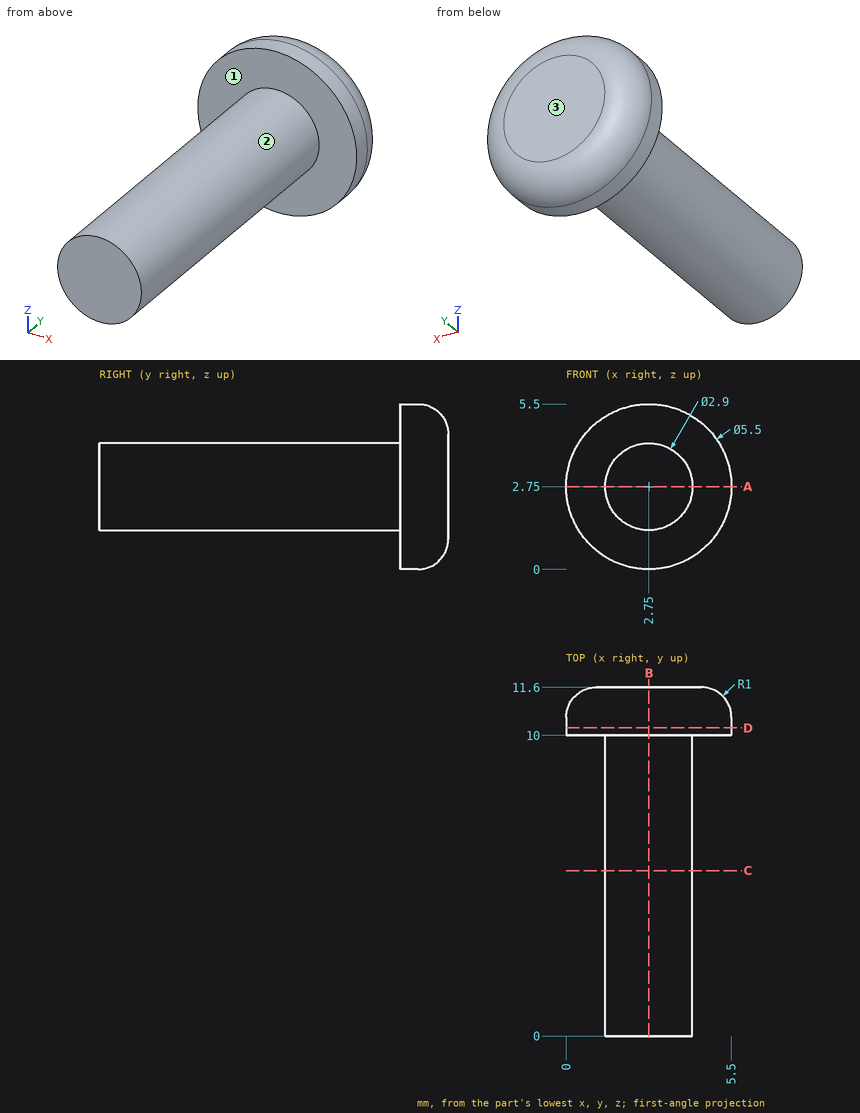
The figure shows three views and two pictorial views of one solid part (mm, origin at its lowest corner). Answer the questions. Give positions to 0.01 mm unless a question says otherwise; leave off trailing zeros. Loops run counter-clockwise (first coordinate to the right, second up) from the corner with the lowest first, then second, coordinate; pieces in that order, holes last. Notation, with made-up numbers: (76, 15.25) - (109, 15.25) arc R26 cw to (109, 52.25) - close; hole circle Ø6 at (35.25, 23.25). An arc over 180 degrees is marked (long way). Use one line per item in the form item = value.
1. Section D-D on y = 10.25 is taken. Give the vertices of the cut face in (x, z).
Calculated:
outline = circle Ø5.5 at (2.75, 2.75)
2. Section A-A on z = 2.75 is taken. Give the vertices of the cut face in (x, y).
Calculated:
outline = (0, 10) - (1.3, 10) - (1.3, 0) - (4.2, 0) - (4.2, 10) - (5.5, 10) - (5.5, 10.6) arc R1 ccw to (4.5, 11.6) - (1, 11.6) arc R1 ccw to (0, 10.6) - close
3. The mould has two halves that part along Y. Classify the marked faces 1, 2 and 3: pulls with the +Y half, pulls with the -Y half, needs draft (parallel to the pull), parting line crosses it, or undercut.
Calculated:
face_1 = pulls with the -Y half
face_2 = needs draft
face_3 = pulls with the +Y half
4. Find the intervals of material crossed by line 1 along X through (y, z) = (0.5, 3.45); line 2 along X through (y, z) = (10.5, 3.8); line 3 along Z through (x, y) = (1.85, 10.25), in increasing order. Write a range as [from, to].
Calculated:
line_1 = [1.48, 4.02]
line_2 = [0.21, 5.29]
line_3 = [0.15, 5.35]
5. Section B-B on x = 2.75 is taken. Give the vertices of the cut face in (y, z), then the cut area to 3 significant figures.
Calculated:
outline = (0, 1.3) - (10, 1.3) - (10, 0) - (10.6, 0) arc R1 ccw to (11.6, 1) - (11.6, 4.5) arc R1 ccw to (10.6, 5.5) - (10, 5.5) - (10, 4.2) - (0, 4.2) - close
area = 37.4 mm^2
6. Section C-C on y = 5.5 is taken. Give the vertices of the cut face in (x, z), then the cut area to 3 significant figures.
Calculated:
outline = circle Ø2.9 at (2.75, 2.75)
area = 6.61 mm^2
7. Given pin 1 Ø1.5 at (y, z) = (4.5, 3) entering from +X, flat-ended and moving along its own axis, determine where the tip first touches the part or whether it passes through.
Calculated:
pin_1 = 4.2
